Work out the finished part from the listing and answer in its coordinate system (mm). Face numbers are marked on the shaded views. A direction names the side the tool comes from. Coordinates: 2 decimals unless noted, no trailing zeros. Order: outer loops, then holes, each group sorted by start corner. A loop starts at its lowest first (then second) coordinate and runs counter-clockwise, first axis right, second up. Notation, with made-up numbers: M 59,42 L 90,42 A9 ccw 90,51 Z; hole C 13.5,73.5 d3. An arc over 180 degrees is marked long. Use a Markdown table: item, result.
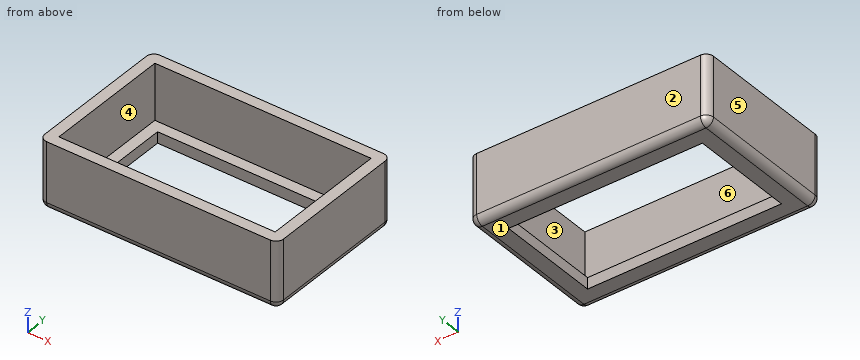
from build123d import *

# Parameters (mm, degrees)
SKETCH1_W           = 16.256
SKETCH1_H           = 10.16
SKETCH1_W_2         = 13.208
SKETCH1_H_2         = 7.112
BOSS_EXTRUDE1_DEPTH = 4.572
SKETCH2_W           = 14.732
SKETCH2_H           = 8.636
CUT_EXTRUDE1_DEPTH  = 3.81
FILLET1_R           = 0.508


with BuildPart() as part:
    # Sketch1 → Boss-Extrude1 (new body)
    with BuildSketch(Plane.XY):
        with Locations((22.86, -62.992)):
            Rectangle(SKETCH1_W, SKETCH1_H)
        with Locations((22.86, -62.992)):
            Rectangle(SKETCH1_W_2, SKETCH1_H_2, mode=Mode.SUBTRACT)
    extrude(amount=-BOSS_EXTRUDE1_DEPTH)

    # Sketch2 → Cut-Extrude1 (cut)
    with BuildSketch(Plane.XY):
        with Locations((22.86, -62.992)):
            Rectangle(SKETCH2_W, SKETCH2_H)
    extrude(amount=-CUT_EXTRUDE1_DEPTH, mode=Mode.SUBTRACT)

    # Fillet1
    fillet1_edges = [part.edges().sort_by_distance(p)[0] for p in [
        (14.732, -62.992, -4.572),
        (22.86, -68.072, -4.572),
        (30.988, -62.992, -4.572),
        (22.86, -57.912, -4.572),
        (30.988, -68.072, -2.286),
        (14.732, -68.072, -2.286),
        (14.732, -57.912, -2.286),
        (30.988, -57.912, -2.286),
    ]]
    fillet(fillet1_edges, radius=FILLET1_R)


solid = part.part
1. Section D-D on y = -59.25 is taken. Determine the outline of the cut face in (x, z), then the cut area to 3 significant figures.
Answers below:
| item | result |
|---|---|
| outline | M 14.73,-4.06 A0.51 ccw 15.24,-4.57 L 30.48,-4.57 A0.51 ccw 30.99,-4.06 L 30.99,0 L 30.23,0 L 30.23,-3.81 L 15.49,-3.81 L 15.49,0 L 14.73,0 Z |
| area | 18.1 mm² |
2. Section C-C on y = -61 is taken. Determine the outline of the cut face in (x, z), then the cut area to 3 significant figures.
Answers below:
| item | result |
|---|---|
| outline | M 14.73,-4.06 A0.51 ccw 15.24,-4.57 L 16.26,-4.57 L 16.26,-3.81 L 15.49,-3.81 L 15.49,0 L 14.73,0 Z; M 29.46,-4.57 L 30.48,-4.57 A0.51 ccw 30.99,-4.06 L 30.99,0 L 30.23,0 L 30.23,-3.81 L 29.46,-3.81 Z |
| area | 8.02 mm² |
3. Section B-B on x = 24 is taken. Determine the outline of the cut face in (y, z), then the cut area to 3 significant figures.
Answers below:
| item | result |
|---|---|
| outline | M -68.07,-4.06 A0.51 ccw -67.56,-4.57 L -66.55,-4.57 L -66.55,-3.81 L -67.31,-3.81 L -67.31,0 L -68.07,0 Z; M -59.44,-4.57 L -58.42,-4.57 A0.51 ccw -57.91,-4.06 L -57.91,0 L -58.67,0 L -58.67,-3.81 L -59.44,-3.81 Z |
| area | 8.02 mm² |
4. For the marked faces 5 and 6, determine the directions among +Z, -Z, +X, -X, +Y, -Y from which every point of the face is accessible in a straight line to the end or side of a thin tool.
Answers below:
| item | result |
|---|---|
| face 5 | +Z, -Z, -X, +Y, -Y |
| face 6 | +Z |
5. Find the intervals of material crossed by probe 1 along Y at (x, z) = (26.75, -3.75); probe 2 along X at (y, z) = (-62, -0.15); probe 3 along Y at (x, z) = (25.25, -4.1), in increasing order.
Answers below:
| item | result |
|---|---|
| probe 1 | -68.07 to -67.31, -58.67 to -57.91 |
| probe 2 | 14.73 to 15.49, 30.23 to 30.99 |
| probe 3 | -68.07 to -66.55, -59.44 to -57.91 |
6. For a pull along Y with two mould halves and no side action, classify the marked faces 1, 2, 3 and 4 as +Y half, -Y half, draft (parallel to the pull), parting line (faces both ways), or undercut.
Answers below:
| item | result |
|---|---|
| face 1 | draft |
| face 2 | +Y half |
| face 3 | undercut |
| face 4 | undercut |
7. Section A-A on z = -1.75 is taken. Determine the outline of the cut face in (x, y).
Answers below:
| item | result |
|---|---|
| outline | M 14.73,-67.56 A0.51 ccw 15.24,-68.07 L 30.48,-68.07 A0.51 ccw 30.99,-67.56 L 30.99,-58.42 A0.51 ccw 30.48,-57.91 L 15.24,-57.91 A0.51 ccw 14.73,-58.42 Z; hole M 15.49,-67.31 L 30.23,-67.31 L 30.23,-58.67 L 15.49,-58.67 Z |
